from build123d import *

# Parameters (mm, degrees)
SKETCH1_W            = 140
SKETCH1_H            = 150
SKETCH1_W_2          = 100.689655172
SKETCH1_H_2          = 60
BOSS_EXTRUDE1_DEPTH  = 30
CUT_EXTRUDE1_DEPTH   = 300
SKETCH11_W           = 140
SKETCH11_H           = 11.715455608
BOSS_EXTRUDE2_DEPTH  = 10
SKETCH3_R            = 3
CUT_EXTRUDE2_DEPTH   = 100
SKETCH4_R            = 7
CUT_EXTRUDE3_DEPTH   = 70
LPATTERN1_COUNT      = 3
LPATTERN1_PITCH      = 40
SKETCH5_R            = 2.238650571
CUT_EXTRUDE4_DEPTH   = 100
SKETCH6_R            = 4.368973
CUT_EXTRUDE5_DEPTH   = 25
LPATTERN2_COUNT      = 2
LPATTERN2_PITCH      = 20
LPATTERN2_COUNT_DIR2 = 2
LPATTERN2_PITCH_DIR2 = 120
SKETCH7_R            = 2.900161541
CUT_EXTRUDE6_DEPTH   = 40
SKETCH8_R            = 5.870976625
CUT_EXTRUDE7_DEPTH   = 25
LPATTERN3_COUNT      = 4
LPATTERN3_PITCH      = 40
LPATTERN3_COUNT_DIR2 = 2
LPATTERN3_PITCH_DIR2 = 80
SKETCH9_R            = 3.381759822
CUT_EXTRUDE8_DEPTH   = 100
CUT_EXTRUDE9_START   = -10
SKETCH10_R           = 6.982534733
CUT_EXTRUDE9_DEPTH   = 20
LPATTERN4_COUNT      = 2
LPATTERN4_PITCH      = 120
CHAMFER1_SIZE        = 5
SKETCH16_W           = 13.0342626
SKETCH16_H           = 10.99288792
CUT_EXTRUDE13_DEPTH  = 20
SKETCH17_R           = 2.765660559
CUT_EXTRUDE14_DEPTH  = 15
LPATTERN6_COUNT      = 4
LPATTERN6_PITCH      = 40


with BuildPart() as part:
    # Sketch1 → Boss-Extrude1 (new body)
    with BuildSketch(Plane.XY):
        with Locations((6.896551724, 31.293103448)):
            Rectangle(SKETCH1_W, SKETCH1_H)
        with Locations((6.551724138, 1.293103448)):
            Rectangle(SKETCH1_W_2, SKETCH1_H_2, mode=Mode.SUBTRACT)
    extrude(amount=BOSS_EXTRUDE1_DEPTH)

    # Sketch2 → Cut-Extrude1 (cut)
    with BuildSketch(Plane.ZY.offset(63.103448276)):
        Polygon((30, 40.467146905), (23.720048633, 36.378281812), (23.720048633, 33.58866414), (30, 31.544440585), align=None)
    cut_extrude1 = extrude(amount=-CUT_EXTRUDE1_DEPTH, mode=Mode.SUBTRACT)

    # Sketch11 → Boss-Extrude2 (add)
    with BuildSketch(Plane.XY.offset(30)):
        with Locations((6.896551724, 46.324874709)):
            Rectangle(SKETCH11_W, SKETCH11_H)
    boss_extrude2 = extrude(amount=BOSS_EXTRUDE2_DEPTH)

    # Mirror1: Cut-Extrude1, Boss-Extrude2 across plane
    add(cut_extrude1.mirror(Plane(origin=(0, 11.293103448, 0), x_dir=(0, 0, 1), z_dir=(0, -1, 0))), mode=Mode.SUBTRACT)
    add(boss_extrude2.mirror(Plane(origin=(0, 11.293103448, 0), x_dir=(0, 0, 1), z_dir=(0, -1, 0))))

    # Sketch3 → Cut-Extrude2 (cut)
    with BuildSketch(Plane(origin=(0, 106.293103448, 0), x_dir=(1, 0, 0), z_dir=(0, 1, 0))):
        with Locations(Location((-29.404551137, -15.436210525, 0), (0, 0, 270))):
            Circle(SKETCH3_R)
    cut_extrude2 = extrude(amount=-CUT_EXTRUDE2_DEPTH, mode=Mode.SUBTRACT)

    # Sketch4 → Cut-Extrude3 (cut)
    with BuildSketch(Plane(origin=(0, 106.293103448, 0), x_dir=(1, 0, 0), z_dir=(0, 1, 0))):
        with Locations(Location((-29.404551137, -15.436210525, 0), (0, 0, 270))):
            Circle(SKETCH4_R)
    cut_extrude3 = extrude(amount=-CUT_EXTRUDE3_DEPTH, mode=Mode.SUBTRACT)

    # LPattern1: Cut-Extrude2, Cut-Extrude3 ×3
    with Locations(*[(i * LPATTERN1_PITCH, 0, 0) for i in range(1, LPATTERN1_COUNT)]):
        add(cut_extrude2, mode=Mode.SUBTRACT)
        add(cut_extrude3, mode=Mode.SUBTRACT)

    # Sketch5 → Cut-Extrude4 (cut)
    with BuildSketch(Plane(origin=(0, 0, 0), x_dir=(-1, 0, 0), z_dir=(0, 0, -1))):
        with Locations((53.103448276, -18.706896552)):
            Circle(SKETCH5_R)
    cut_extrude4 = extrude(amount=-CUT_EXTRUDE4_DEPTH, mode=Mode.SUBTRACT)

    # Sketch6 → Cut-Extrude5 (cut)
    with BuildSketch(Plane(origin=(0, 0, 0), x_dir=(-1, 0, 0), z_dir=(0, 0, -1))):
        with Locations((53.103448276, -18.706896552)):
            Circle(SKETCH6_R)
    cut_extrude5 = extrude(amount=-CUT_EXTRUDE5_DEPTH, mode=Mode.SUBTRACT)

    # LPattern2: Cut-Extrude4, Cut-Extrude5 2 × 2
    with Locations(*[(j * LPATTERN2_PITCH_DIR2, i * LPATTERN2_PITCH, 0) for i in range(LPATTERN2_COUNT) for j in range(LPATTERN2_COUNT_DIR2) if (i, j) != (0, 0)]):
        add(cut_extrude4, mode=Mode.SUBTRACT)
        add(cut_extrude5, mode=Mode.SUBTRACT)

    # Sketch7 → Cut-Extrude6 (cut)
    with BuildSketch(Plane(origin=(0, 0, 0), x_dir=(-1, 0, 0), z_dir=(0, 0, -1))):
        with Locations((51.00310189, 51.293103448)):
            Circle(SKETCH7_R)
    cut_extrude6 = extrude(amount=-CUT_EXTRUDE6_DEPTH, mode=Mode.SUBTRACT)

    # Sketch8 → Cut-Extrude7 (cut)
    with BuildSketch(Plane(origin=(0, 0, 0), x_dir=(-1, 0, 0), z_dir=(0, 0, -1))):
        with Locations((51.00310189, 51.293103448)):
            Circle(SKETCH8_R)
    cut_extrude7 = extrude(amount=-CUT_EXTRUDE7_DEPTH, mode=Mode.SUBTRACT)

    # LPattern3: Cut-Extrude6, Cut-Extrude7 4 × 2
    with Locations(*[(i * LPATTERN3_PITCH, -j * LPATTERN3_PITCH_DIR2, 0) for i in range(LPATTERN3_COUNT) for j in range(LPATTERN3_COUNT_DIR2) if (i, j) != (0, 0)]):
        add(cut_extrude6, mode=Mode.SUBTRACT)
        add(cut_extrude7, mode=Mode.SUBTRACT)

    # Sketch9 → Cut-Extrude8 (cut)
    with BuildSketch(Plane(origin=(0, 0, 0), x_dir=(-1, 0, 0), z_dir=(0, 0, -1))):
        with Locations((-66.896551724, 66.293103448)):
            Circle(SKETCH9_R)
    cut_extrude8 = extrude(amount=-CUT_EXTRUDE8_DEPTH, mode=Mode.SUBTRACT)

    # Sketch10 → Cut-Extrude9 (cut)
    with BuildSketch(Plane.XY.offset(30).offset(CUT_EXTRUDE9_START)):
        with Locations((66.896551724, 66.293103448)):
            Circle(SKETCH10_R)
    cut_extrude9 = extrude(amount=-CUT_EXTRUDE9_DEPTH, mode=Mode.SUBTRACT)

    # LPattern4: Cut-Extrude8, Cut-Extrude9 ×2
    with Locations(*[(-i * LPATTERN4_PITCH, 0, 0) for i in range(1, LPATTERN4_COUNT)]):
        add(cut_extrude8, mode=Mode.SUBTRACT)
        add(cut_extrude9, mode=Mode.SUBTRACT)

    # Chamfer1
    chamfer1_edges = [part.edges().sort_by_distance(p)[0] for p in [
        (6.896551724, 106.293103448, 30),
        (6.896551724, 106.293103448, 0),
    ]]
    chamfer(chamfer1_edges, length=CHAMFER1_SIZE)

    # Sketch16 → Cut-Extrude13 (cut)
    with BuildSketch(Plane(origin=(0, 0, 0), x_dir=(-1, 0, 0), z_dir=(0, 0, -1))):
        with Locations((-66.003847549, 93.127101144)):
            Rectangle(SKETCH16_W, SKETCH16_H)
    cut_extrude13 = extrude(amount=-CUT_EXTRUDE13_DEPTH, mode=Mode.SUBTRACT)

    # Sketch17 → Cut-Extrude14 (cut)
    with BuildSketch(Plane(origin=(0, 106.293103448, 0), x_dir=(1, 0, 0), z_dir=(0, 1, 0))):
        with Locations(Location((66.162561207, -15.398222954, 0), (0, 0, 270))):
            Circle(SKETCH17_R)
    cut_extrude14 = extrude(amount=-CUT_EXTRUDE14_DEPTH, mode=Mode.SUBTRACT)

    # LPattern6: Cut-Extrude13, Cut-Extrude14 ×4
    with Locations(*[(-i * LPATTERN6_PITCH, 0, 0) for i in range(1, LPATTERN6_COUNT)]):
        add(cut_extrude13, mode=Mode.SUBTRACT)
        add(cut_extrude14, mode=Mode.SUBTRACT)


solid = part.part
Verification items for the finished model (mm, model axes). A direction names the side the tool comes from. Give positions to 0.01 mm unless a question says otherwise; leave off trailing zeros. Loops run counter-clockwise (first coordinate to the right, second up) from the corner with the lowest first, then second, coordinate; pieces in that order, holes last. Notation, with made-up numbers: (-8, 74.25) - (1, 74.25) arc R26 cw to (1, 89.25) - close; hole circle Ø3 at (32.5, 75). An arc over 180 degrees is marked (long way). Write each question's results on one line, items separated by ' | '.
1) Depth check by flat-ended pin: P1, Ø9.5, axis at x = -51, y = -28.71, coming from the -Z side; P2, Ø3.5, axis at x = 66, y = 92, coming from the -Z side; P3, Ø3, axis at x = -31, z = 34, coming from the +Y side. Enter the tip coordinate at first touch or a pass-through.
Solution:
P1: z = 25 | P2: z = 20 | P3: y = 52.18
2) Mould release check, pull along X, two halves, no side actions. Record for faces 4 (the flat face through (6, 40.467, 35)), 5 (the cylindrical face through (-54.184, -14.474, 12.325)): pulls with the +X half, pulls with the -X half, needs draft (parallel to the pull), parting line crosses it, or undercut.
Solution:
face 4: needs draft | face 5: undercut
3) Material ranges on L1, parallel to Y at x = -37.5, z = 38.5; L2, parallel to Y at x = 18.5, z = 21; L3, parallel to X at y = 4, z = 26, recorded low to high. Write a range as from..to.
Solution:
L1: -29.6..-17.88, 40.47..52.18 | L2: -43.71..-28.71, 31.29..106.29 | L3: -63.1..-43.79, 56.9..76.9
4) Sectioned sample at D-D on z = 14.5. Count the separate pieces of the cut face and the enclosed holes in it, plus the area to 3 significant figures.
Solution:
separate pieces: 3 | enclosed holes: 10 | area: 9,920 mm2
5) Tool access check on faces 1 (the flat face through (6, -17.881, 35)), 2 (the flat face through (49, 52.183, 35)), 3 (the flat face through (-29, -28.707, 15)). Record the directions out of +Z, -Z, +X, -X, +Y, -Y that give a thin tool (end or side, any length) a straight path to the whole face; none if there is none.
Solution:
face 1: +Z, +X, -X | face 2: +Z, +X, -X, +Y | face 3: -Z
6) Sectioned sample at C-C on y = 38.5. Record the boundary of the cut face in (x, z), plus the area to 3 significant figures.
Solution:
outline: (-63.1, 0) - (76.9, 0) - (76.9, 26.98) - (-63.1, 26.98) - close; hole circle Ø14 at (-29.4, 15.44); hole circle Ø14 at (10.6, 15.44); hole circle Ø14 at (50.6, 15.44) | area: 3,320 mm2
7) Sectioned sample at B-B on x = -41.5. Record the boundary of the cut face in (y, z), plus the area to 3 significant figures.
Solution:
outline: (-43.71, 0) - (-28.71, 0) - (-28.71, 30) - (-17.88, 30) - (-17.88, 40) - (-29.6, 40) - (-29.6, 30) - (-43.71, 30) - close; (31.29, 0) - (101.29, 0) - (106.29, 5) - (106.29, 25) - (101.29, 30) - (52.18, 30) - (52.18, 40) - (40.47, 40) - (40.47, 30) - (36.38, 23.72) - (33.59, 23.72) - (31.54, 30) - (31.29, 30) - close | area: 2,870 mm2
8) Sectioned sample at A-A on z = 34. Record the boundary of the cut face in (x, y), plus the area to 3 significant figures.
Solution:
outline: (-63.1, -29.6) - (-53.76, -29.6) arc R2.9 cw (long way) to (-48.24, -29.6) - (-13.76, -29.6) arc R2.9 cw (long way) to (-8.24, -29.6) - (26.24, -29.6) arc R2.9 cw (long way) to (31.76, -29.6) - (66.24, -29.6) arc R2.9 cw (long way) to (71.76, -29.6) - (76.9, -29.6) - (76.9, -17.88) - (68.98, -17.88) arc R2.24 cw (long way) to (64.82, -17.88) - (-51.02, -17.88) arc R2.24 cw (long way) to (-55.18, -17.88) - (-63.1, -17.88) - close; (-63.1, 40.47) - (76.9, 40.47) - (76.9, 52.18) - (71.76, 52.18) arc R2.9 cw (long way) to (66.24, 52.18) - (31.76, 52.18) arc R2.9 cw (long way) to (26.24, 52.18) - (-8.24, 52.18) arc R2.9 cw (long way) to (-13.76, 52.18) - (-48.24, 52.18) arc R2.9 cw (long way) to (-53.76, 52.18) - (-63.1, 52.18) - close | area: 3,110 mm2
